The listing builds one solid part. Answer for the finished solid, in the listing's coordinates (mm). Face numbers are marked on the shaded views. A direction names the side the tool comes from. Round coordinates to 2 decimals unless told otherwise and drop trailing zeros. Write each loop counter-clockwise with the first axis right and the second up, starting at its lowest first coordinate (ties: lowest second). Pieces come first, ordered by that corner, then holes. Notation, with made-up numbers: (13.5, -24.75) - (18.5, -24.75) arc R13 ccw to (18.5, -2.75) - close; hole circle Ø11 at (-27.5, -27.75). An arc over 180 degrees is marked (long way). Answer as CSV lines item,"result". Start each with the question number.
Item 1: For a pull along Y with two mould halves and no side action, classify the marked faces 3, 4 and 5 as pulls with the +Y half, pulls with the -Y half, needs draft (parallel to the pull), parting line crosses it, or undercut.
Item 2: Straight lines are drawn through the part: line 1 along Z through (x, y) = (8.5, 9.75); line 2 along Y through (x, z) = (15.5, -8.25); line 3 along Z through (x, y) = (3.5, 7.25). For each, find the intervals that lie inside material, in ascending order. Write a range as [from, to].
Item 3: Which of the six approach directions +Z, -Z, +X, -X, +Y, -Y give full straight-line access (tool end or side, diameter ignored) to the marked faces 1 and 2?
Item 4: A cutting plane is placed at C-C on y = 0. Determine the outline of the cut face in (x, z) (3 decimals), and give its area (3 significant figures).
Item 5: Flat-ended cylindrical pins translate along their axes: pin 1 (8 mm diameter, centred on x = 6.5, z = 8.5, fed in from -Y); pin 2 (8 mm diameter, centred on x = 2.5, z = -4.5, fed in from +Y); pin 3 (2 mm diameter, centred on x = 12, y = 3.5, fed in from +Z). Find the tip coordinate at first contact, or state that the pin passes through.
Item 6: A cutting plane is placed at A-A on x = 12.25. Determine the outline of the cut face in (y, z) (3 decimals), and give its area (3 significant figures).
```python
from build123d import *
from OCP.BRepFilletAPI import BRepFilletAPI_MakeChamfer

# Parameters (mm, degrees)
ID_CHAMFER_SIZE   = 0.25
ID_CHAMFER_SIZE2  = 0.307635462
OD_CHAMFER_SIZE   = 0.25
OD_CHAMFER_SIZE2  = 0.275015717
BORE_SLOT_DEPTH   = 25.334248499
CIRPATTERN1_COUNT = 3


with BuildPart() as part:
    # Sketch1 → Revolve1 (revolve)
    with BuildSketch(Plane.XY, mode=Mode.PRIVATE) as revolve1_sk:
        with BuildLine():
            Line((0, 10), (0, 12.593767005))
            Line((0, 12.593767005), (1.5, 12.725))
            Line((1.5, 12.725), (14.88, 12.725))
            Line((14.88, 12.725), (16.38, 12.593767005))
            Line((16.38, 12.593767005), (16.38, 10))
            Line((16.38, 10), (14.38, 9.65))
            Line((14.38, 9.65), (10.88, 9.65))
            ThreePointArc((10.88, 9.65), (10.38, 9.75), (9.88, 9.65))
            Line((9.88, 9.65), (6.5, 9.65))
            ThreePointArc((6.5, 9.65), (6, 9.75), (5.5, 9.65))
            Line((5.5, 9.65), (2, 9.65))
            Line((2, 9.65), (0, 10))
        make_face()
    revolve(revolve1_sk.sketch.rotate(Axis((-2.430533636, 0, 0), (1, 0, 0)), 90), axis=Axis((-2.430533636, 0, 0), (1, 0, 0)))

    # ID Chamfer: one chamfer whose edges measure the first distance from different faces: ONE call of the kernel's chamfer builder (chamfer() names one face for all edges)
    id_chamfer_edges_1 = [part.edges().sort_by_distance(p)[0] for p in [
        (16.38, 0, -10),
    ]]
    id_chamfer_side_1 = [part.faces().sort_by_distance(p)[0] for p in [
        (15.38, 0, -9.825),
    ]]
    id_chamfer_edges_2 = [part.edges().sort_by_distance(p)[0] for p in [
        (0, 0, -10),
    ]]
    id_chamfer_side_2 = [part.faces().sort_by_distance(p)[0] for p in [
        (0, 0, -10.356205522),
    ]]
    id_chamfer = BRepFilletAPI_MakeChamfer(part.part.solid().wrapped)
    for e in id_chamfer_edges_1:
        id_chamfer.Add(ID_CHAMFER_SIZE, ID_CHAMFER_SIZE2, e.wrapped, id_chamfer_side_1[0].wrapped)  # the first distance lies on this face
    for e in id_chamfer_edges_2:
        id_chamfer.Add(ID_CHAMFER_SIZE, ID_CHAMFER_SIZE2, e.wrapped, id_chamfer_side_2[0].wrapped)  # the first distance lies on this face
    add(Compound.cast(id_chamfer.Shape()), mode=Mode.REPLACE)

    # OD Chamfer: one chamfer whose edges measure the first distance from different faces: ONE call of the kernel's chamfer builder (chamfer() names one face for all edges)
    od_chamfer_edges_1 = [part.edges().sort_by_distance(p)[0] for p in [
        (16.38, 0, -12.593767005),
    ]]
    od_chamfer_side_1 = [part.faces().sort_by_distance(p)[0] for p in [
        (16.38, 0, -10.663840984),
    ]]
    od_chamfer_edges_2 = [part.edges().sort_by_distance(p)[0] for p in [
        (0, 0, -12.593767005),
    ]]
    od_chamfer_side_2 = [part.faces().sort_by_distance(p)[0] for p in [
        (0.75, 0, -12.659383502),
    ]]
    od_chamfer = BRepFilletAPI_MakeChamfer(part.part.solid().wrapped)
    for e in od_chamfer_edges_1:
        od_chamfer.Add(OD_CHAMFER_SIZE, OD_CHAMFER_SIZE2, e.wrapped, od_chamfer_side_1[0].wrapped)  # the first distance lies on this face
    for e in od_chamfer_edges_2:
        od_chamfer.Add(OD_CHAMFER_SIZE, OD_CHAMFER_SIZE2, e.wrapped, od_chamfer_side_2[0].wrapped)  # the first distance lies on this face
    add(Compound.cast(od_chamfer.Shape()), mode=Mode.REPLACE)

    # Sketch2 → Bore Slot (cut, through all)
    with BuildSketch(Plane(origin=(0, 0, 0), x_dir=(0, 0, -1), z_dir=(1, 0, 0))):
        with BuildLine():
            ThreePointArc((-4.075172705, 8.747312011), (-4.9, 8.487048957), (-5.537808064, 7.902859093))
            ThreePointArc((-5.537808064, 7.902859093), (-4.825, 8.357145147), (-4.075172705, 8.747312011))
        make_face()
    bore_slot = extrude(amount=BORE_SLOT_DEPTH, mode=Mode.SUBTRACT)

    # CirPattern1: Bore Slot ×3 about axis
    cirpattern1_axis = Axis((0, 0, 0), (1, 0, 0))
    for i in range(1, CIRPATTERN1_COUNT):
        add(bore_slot.rotate(cirpattern1_axis, i * 360 / CIRPATTERN1_COUNT), mode=Mode.SUBTRACT)


solid = part.part
```
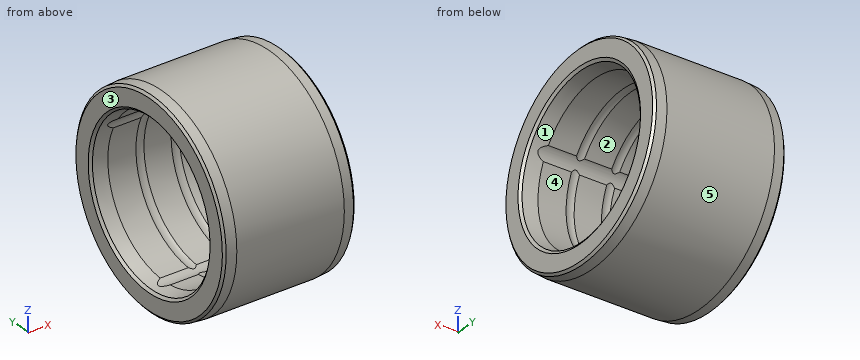
Geometry says:
1,face 3,"needs draft"
1,face 4,"undercut"
1,face 5,"parting line crosses it"
2,line 1,"z = [-8.18, 8.18]"
2,line 2,"y = [-9.62, -5.37], [5.37, 9.62]"
2,line 3,"z = [-10.46, -6.37], [6.37, 10.46]"
3,face 1,"+X"
3,face 2,"+X, -X"
4,outline,"(0, -12.319) - (0.249, -12.616) - (1.5, -12.725) - (14.88, -12.725) - (16.106, -12.618) - (16.38, -12.344) - (16.38, -10.308) - (16.134, -9.957) - (15.237, -9.8) - (1.143, -9.8) - (0.303, -9.947) - (0, -10.25) - close; (0, 10.25) - (0.303, 9.947) - (2, 9.65) - (5.5, 9.65) arc R1.3 cw to (6.5, 9.65) - (9.88, 9.65) arc R1.3 cw to (10.88, 9.65) - (14.38, 9.65) - (16.134, 9.957) - (16.38, 10.308) - (16.38, 12.344) - (16.106, 12.618) - (14.88, 12.725) - (1.5, 12.725) - (0.249, 12.616) - (0, 12.319) - close"
4,area,"96.5 mm^2"
5,pin 1,"stops at y = -11.9"
5,pin 2,"stops at y = 12.72"
5,pin 3,"stops at z = 12.48"
6,outline,"circle Ø25.45 at (0, 0); hole (-8.747, 4.075) arc R9.65 ccw to (-0.844, -9.613) arc R2 ccw to (0.844, -9.613) arc R9.65 ccw to (8.747, 4.075) arc R2 ccw to (7.903, 5.538) arc R9.65 ccw to (-7.903, 5.538) arc R2 ccw to start"
6,area,"216 mm^2"
